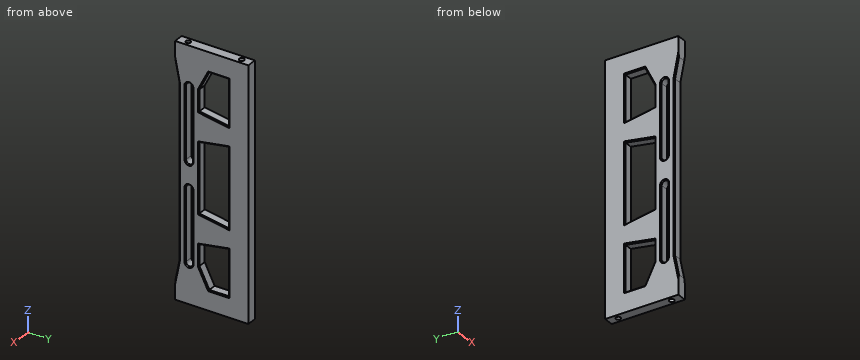
from build123d import *

# Parameters (mm, degrees)
CROQUIS1_W              = 5
CROQUIS1_H              = 10
SALIENTE_EXTRUIR1_DEPTH = 126
SALIENTE_EXTRUIR2_DEPTH = 5
CROQUIS2_R              = 1.25
CORTAR_EXTRUIR1_DEPTH   = 10
CROQUIS3_R              = 1.25
CORTAR_EXTRUIR2_DEPTH   = 10
CHAFL_N1_SIZE           = 0.5


with BuildPart() as part:
    # Croquis1 → Saliente-Extruir1 (new body)
    with BuildSketch(Plane.XY):
        Rectangle(CROQUIS1_W, CROQUIS1_H)
    extrude(amount=SALIENTE_EXTRUIR1_DEPTH)

    # Croquis4 → Saliente-Extruir2 (add)
    with BuildSketch(Plane.ZY.offset(2.5)):
        Polygon((0, -5), (0, -32), (10, -32), (20, -30), (106, -30), (116, -32), (126, -32), (126, -5), (116, -5), (116, -15), (106, -20), (95.375, -20), (92.875, -5), (82.875, -5), (80.375, -20), (45.625, -20), (43.125, -5), (33.125, -5), (30.625, -20), (20, -20), (10, -15), (10, -5), align=None)
        with BuildLine():
            Line((20, -23.25), (56.25, -23.25))
            ThreePointArc((56.25, -23.25), (58, -25), (56.25, -26.75))
            Line((56.25, -26.75), (20, -26.75))
            ThreePointArc((20, -26.75), (18.25, -25), (20, -23.25))
        make_face(mode=Mode.SUBTRACT)
        with BuildLine():
            Line((69.75, -23.25), (106, -23.25))
            ThreePointArc((106, -23.25), (107.75, -25), (106, -26.75))
            Line((106, -26.75), (69.75, -26.75))
            ThreePointArc((69.75, -26.75), (68, -25), (69.75, -23.25))
        make_face(mode=Mode.SUBTRACT)
    extrude(amount=-SALIENTE_EXTRUIR2_DEPTH)

    # Croquis2 → Cortar-Extruir1 (cut)
    with BuildSketch(Plane.XY.offset(126)):
        Circle(CROQUIS2_R)
        with Locations((0, -27)):
            Circle(CROQUIS2_R)
    extrude(amount=-CORTAR_EXTRUIR1_DEPTH, mode=Mode.SUBTRACT)

    # Croquis3 → Cortar-Extruir2 (cut)
    with BuildSketch(Plane(origin=(0, 0, 0), x_dir=(-1, 0, 0), z_dir=(0, 0, -1))):
        Circle(CROQUIS3_R)
        with Locations((0, -27)):
            Circle(CROQUIS3_R)
    extrude(amount=-CORTAR_EXTRUIR2_DEPTH, mode=Mode.SUBTRACT)

    # Chaflán1
    chafl_n1_edges = [part.edges().sort_by_distance(p)[0] for p in [
        (2.5, -5, 104.4375),
        (2.5, -5, 63),
        (2.5, -5, 21.5625),
        (-2.5, -5, 104.4375),
        (-2.5, -5, 63),
        (-2.5, -5, 21.5625),
        (2.5, -10, 10),
        (2.5, -17.5, 15),
        (2.5, -20, 25.3125),
        (2.5, -12.5, 31.875),
        (2.5, -12.5, 44.375),
        (2.5, -20, 63),
        (2.5, -12.5, 81.625),
        (2.5, -12.5, 94.125),
        (2.5, -20, 100.6875),
        (2.5, -17.5, 111),
        (2.5, -10, 116),
        (2.5, -31, 111),
        (2.5, -30, 63),
        (2.5, -31, 15),
        (2.5, -25, 18.25),
        (2.5, -26.75, 38.125),
        (2.5, -25, 58),
        (2.5, -23.25, 38.125),
        (2.5, -25, 68),
        (2.5, -26.75, 87.875),
        (2.5, -25, 107.75),
        (2.5, -23.25, 87.875),
        (-2.5, -31, 15),
        (-2.5, -30, 63),
        (-2.5, -31, 111),
        (-2.5, -10, 116),
        (-2.5, -17.5, 111),
        (-2.5, -20, 100.6875),
        (-2.5, -12.5, 94.125),
        (-2.5, -12.5, 81.625),
        (-2.5, -20, 63),
        (-2.5, -12.5, 44.375),
        (-2.5, -12.5, 31.875),
        (-2.5, -20, 25.3125),
        (-2.5, -17.5, 15),
        (-2.5, -10, 10),
        (-2.5, -25, 68),
        (-2.5, -23.25, 87.875),
        (-2.5, -25, 107.75),
        (-2.5, -26.75, 87.875),
        (-2.5, -25, 18.25),
        (-2.5, -23.25, 38.125),
        (-2.5, -25, 58),
        (-2.5, -26.75, 38.125),
    ]]
    chamfer(chafl_n1_edges, length=CHAFL_N1_SIZE)


solid = part.part
For this review, take the finished solid that the model builds, in its own axes (mm). Give positions to 0.01 mm unless a question says otherwise; leave off trailing zeros. Order: outer loops, then holes, each group sorted by start corner. A loop starts at its lowest first (then second) coordinate and runs counter-clockwise, first axis right, second up. Notation, with made-up numbers: (-31, -7.5) - (-19, -7.5) arc R17 cw to (-19, 0.5) - close; hole circle Ø3 at (62.5, 79). An arc over 180 degrees is marked (long way). Answer as a JSON object with one key per item and string values. Group by question number.
Item 1: Wall thickness on line 1 along Y through (x, z) = (1, 96.5); line 2 along Y through (x, z) = (0, 6); line 3 along Z through (x, y) = (-1.3, -25): over which ranges is each line inside the solid? List them lowest first.
Item 2: Clearance check with flat-ended pins moving along their axes: pin 1 Ø2 at (x, y) = (0, 0.5) entering from +Z; pin 2 Ø2 at (x, z) = (-0.5, 64) entering from -Y; pin 3 Ø3 at (x, z) = (0.5, 16) entering from -Y; pin 4 Ø0.8 at (x, y) = (-0.5, -0.5) entering from -Z. State where each tip first meets the part, or that it passes through.
Item 3: Take a section at A-A on y = -7. Give the boundary of the cut face in (x, z).
Item 4: Take a section at D-D on y = 0. Give the boundary of the cut face in (x, z).
Item 5: Take a section at B-B on z = 12.5. Give the boundary of the cut face in (x, y), and give its area (3 significant figures).
Item 6: Take a section at C-C on x = 0. Give the number of separate pieces and of enclosed holes in the cut face, and give its area (3 significant figures).
Reported:
{
 "1": {"line 1": "-30 to -26.75, -23.25 to -20, -5 to 5", "line 2": "-32 to -28.25, -25.75 to -1.25, 1.25 to 5", "line 3": "0 to 18.25, 58 to 68, 107.75 to 126"},
 "2": {"pin 1": "z = 126", "pin 2": "y = -30", "pin 3": "y = -31.1", "pin 4": "z = 10"},
 "3": {"outline": "(-2.5, 0) - (2.5, 0) - (2.5, 9.5) - (2, 10) - (-2, 10) - (-2.5, 9.5) - close; (-2.5, 33.3) - (-2, 32.79) - (2, 32.79) - (2.5, 33.3) - (2.5, 42.95) - (2, 43.46) - (-2, 43.46) - (-2.5, 42.95) - close; (-2.5, 83.05) - (-2, 82.54) - (2, 82.54) - (2.5, 83.05) - (2.5, 92.7) - (2, 93.21) - (-2, 93.21) - (-2.5, 92.7) - close; (-2.5, 116.5) - (-2, 116) - (2, 116) - (2.5, 116.5) - (2.5, 126) - (-2.5, 126) - close"},
 "4": {"outline": "(-2.5, 0) - (-1.25, 0) - (-1.25, 10) - (1.25, 10) - (1.25, 0) - (2.5, 0) - (2.5, 126) - (1.25, 126) - (1.25, 116) - (-1.25, 116) - (-1.25, 126) - (-2.5, 126) - close"},
 "5": {"outline": "(-2.5, -30.99) - (-2, -31.5) - (2, -31.5) - (2.5, -30.99) - (2.5, -16.81) - (2, -16.25) - (-2, -16.25) - (-2.5, -16.81) - close; (-2.5, -4.5) - (-2, -5) - (2, -5) - (2.5, -4.5) - (2.5, 5) - (-2.5, 5) - close", "area": "125 mm^2"},
 "6": {"separate pieces": "1", "enclosed holes": "5", "area": "2,930 mm^2"}
}
